Input: part model. Units: mm. Frame: model coordinates. Face numbers are marked on the shaded views. Coordinates: 2 decimals unless noted, no trailing zeros. Write each loop counter-clockwise with the first axis right and the second up, starting at its lowest first coordinate (ties: lowest second). Pieces come first, ordered by that corner, then holes.
Autodesk Inventor part; units mm, degrees
ref_plane "YZ Plane" through (0, 0, 0) normal (1, 0, 0) x (0, 1, 0)
ref_plane "XZ Plane" through (0, 0, 0) normal (0, 1, 0) x (-1, 0, 0)
ref_plane "XY Plane" through (0, 0, 0) normal (0, 0, 1) x (1, 0, 0)
sketch "Sketch1" plane through (0, 0, 0) normal (1, 0, 0) x (0, 1, 0)
  line L0 (0, 0) -> (0, -1154)
  line L1 (0, -1154) -> (265, -1154)
  line L2 (265, -1154) -> (265, 0)
  line L3 (265, 0) -> (0, 0)
  line L4 (265, 0) -> (290, 0)
  line L5 (290, 0) -> (290, -40)
  line L6 (290, -40) -> (275, -40)
  line L7 (275, -40) -> (275, -1114)
  line L8 (275, -1114) -> (290, -1114)
  line L9 (290, -1114) -> (290, -1154)
  line L10 (265, -1154) -> (290, -1154)
  dimension "d16" = 530
  dimension "d17" = 550
  dimension "d18" = 580
  dimension "d19" = 40
  dimension "d20" = 40
  dimension "d21" = 1154
revolve "Revolution1" add sketch "Sketch1" angle 360 about axis through (0, 0, 0) along (0, 0, -1) contours L4 L5 L6 L7 L8 L9 L10 L2
properties part number "DiscoCorpoTurbina3" material "Steel, Alloy"
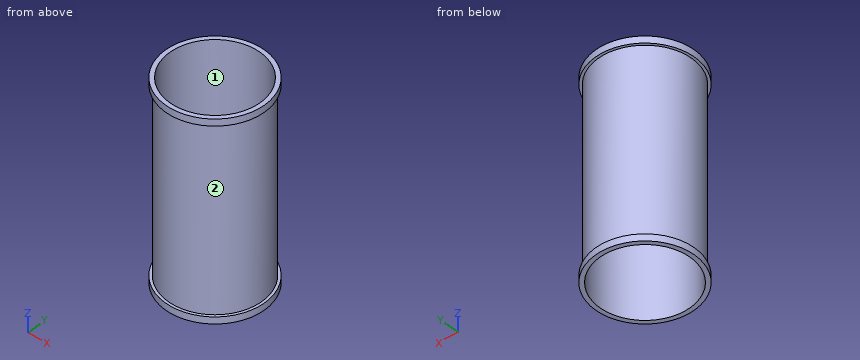
Item 1: Pull-direction query (Z, two-part tool) for the marked faces 1 and 2; classes: released by +Z, released by -Z, zero draft, split by the parting line, or undercut.
Item 2: Section query A-A, the plane x = 0. Return loops of the section in (y, z).
Item 3: Material intervals for line 1 (X direction, y = 0, z = -236.5); line 2 (Z direction, x = 242, y = -147); line 3 (X direction, y = 78.5, z = -814), sorted ascending.
Item 4: Section query B-B, the plane y = 27. Return loops of the section in (x, z), then the cut area to 3 significant figures.
Item 5: Section query C-C, the plane z = -86. Return loops of the section in (x, y).
Item 6: Pin query (flat end, axial travel): pin 1 Ø1 at (x, z) = (-163.5, -283.5) entering from -Y; pin 2 Ø3 at (x, z) = (-181, -142) entering from -Y; pin 3 Ø4 at (y, z) = (-32.5, -515) entering from +X. Return the tip coordinate at first contact, or that it passes through.
The answers:
1. face 1: zero draft
1. face 2: undercut
2. outline: (-290, -1154) - (-265, -1154) - (-265, 0) - (-290, 0) - (-290, -40) - (-275, -40) - (-275, -1114) - (-290, -1114) - close; (265, -1154) - (290, -1154) - (290, -1114) - (275, -1114) - (275, -40) - (290, -40) - (290, 0) - (265, 0) - close
3. line 1: x = -275 to -265, 265 to 275
3. line 2: z = -1154 to -1114, -40 to 0
3. line 3: x = -263.56 to -253.11, 253.11 to 263.56
4. outline: (-288.74, -1154) - (-263.62, -1154) - (-263.62, 0) - (-288.74, 0) - (-288.74, -40) - (-273.67, -40) - (-273.67, -1114) - (-288.74, -1114) - close; (263.62, -1154) - (288.74, -1154) - (288.74, -1114) - (273.67, -1114) - (273.67, -40) - (288.74, -40) - (288.74, 0) - (263.62, 0) - close
4. area: 25,600 mm2
5. outline: circle Ø550 at (0, 0); hole circle Ø530 at (0, 0)
6. pin 1: stops at y = -221.49
6. pin 2: stops at y = -208.34
6. pin 3: stops at x = 273.3
